from build123d import *

# Parameters (mm, degrees)
PAD_DEPTH       = 20
SKETCH001_R     = 1.5
POCKET_DEPTH    = 50.001
SKETCH002_R     = 2.25
POCKET001_DEPTH = 10.001
SKETCH003_R     = 3.5
POCKET002_DEPTH = 2
PAD001_DEPTH    = 10
SKETCH006_W     = 17
SKETCH006_H     = 7
PAD002_DEPTH    = 36
SKETCH007_W     = 17
SKETCH007_H     = 13
PAD003_DEPTH    = 4
FILLET_R        = 3.5
FILLET001_R     = 3.5
FILLET002_R     = 6
FILLET003_R     = 6
FILLET004_R     = 5
FILLET005_R     = 5
FILLET006_R     = 5
FILLET007_R     = 2
FILLET008_R     = 2
POCKET003_START = -3
SKETCH008_W     = 1.5
SKETCH008_H     = 7
POCKET003_DEPTH = 32


with BuildPart() as part:
    # Sketch → Pad (new body)
    with BuildSketch(Plane.XY):
        Polygon((0, 50), (0, 0), (178, 0), (178, 10), (10, 10), (10, 50), align=None)
    extrude(amount=PAD_DEPTH)

    # Sketch001 (on Face2 of Pad) → Pocket (cut, through all)
    with BuildSketch(Plane.XZ):
        with Locations((117.5, 10)):
            Circle(SKETCH001_R)
        with Locations((167.5, 10)):
            Circle(SKETCH001_R)
    extrude(amount=-POCKET_DEPTH, mode=Mode.SUBTRACT)

    # Sketch002 (on Face6 of Pocket) → Pocket001 (cut, through all)
    with BuildSketch(Plane.YZ.offset(10)):
        with Locations((19.428571, 10)):
            Circle(SKETCH002_R)
        with Locations((36.571429, 10)):
            Circle(SKETCH002_R)
    extrude(amount=-POCKET001_DEPTH, mode=Mode.SUBTRACT)

    # Sketch003 (on Face5 of Pocket001) → Pocket002 (cut)
    with BuildSketch(Plane.XZ):
        with Locations((117.5, 10)):
            Circle(SKETCH003_R)
        with Locations((167.5, 10)):
            Circle(SKETCH003_R)
    extrude(amount=-POCKET002_DEPTH, mode=Mode.SUBTRACT)

    # Sketch004 (on Face10 of Pocket002) → Pad001 (join)
    with BuildSketch(Plane(origin=(0, 10, 0), x_dir=(-1, 0, 0), z_dir=(0, 1, 0))):
        Polygon((-35.5, 20), (-35.5, 51.5), (-52.5, 51.5), (-178, 20), (-149.246042, 20), (-52.5, 44.282871), (-52.5, 20), align=None)
        Polygon((-52.5, 0), (-52.5, -24.282871), (-149.246042, 0), (-178, 0), (-52.5, -31.5), (-35.5, -31.5), (-35.5, 0), align=None)
    extrude(amount=-PAD001_DEPTH)

    # Sketch006 (on Face15 of Pad001) → Pad002 (join)
    with BuildSketch(Plane.XZ):
        with Locations((44, 55)):
            Rectangle(SKETCH006_W, SKETCH006_H)
        with Locations((44, -35)):
            Rectangle(SKETCH006_W, SKETCH006_H)
    extrude(amount=-PAD002_DEPTH)

    # Sketch007 (on Face31 of Pad002) → Pad003 (join)
    with BuildSketch(Plane(origin=(0, 36, 0), x_dir=(-1, 0, 0), z_dir=(0, 1, 0))):
        with Locations((-44, -32)):
            Rectangle(SKETCH007_W, SKETCH007_H)
        with Locations((-44, 52)):
            Rectangle(SKETCH007_W, SKETCH007_H)
    extrude(amount=PAD003_DEPTH)

    # Fillet
    fillet_edges = [part.edges().sort_by_distance(p)[0] for p in [
        (44, 40, 45.5),
    ]]
    fillet(fillet_edges, radius=FILLET_R)

    # Fillet001
    fillet001_edges = [part.edges().sort_by_distance(p)[0] for p in [
        (44, 40, -25.5),
    ]]
    fillet(fillet001_edges, radius=FILLET001_R)

    # Fillet002
    fillet002_edges = [part.edges().sort_by_distance(p)[0] for p in [
        (44, 40, 58.5),
    ]]
    fillet(fillet002_edges, radius=FILLET002_R)

    # Fillet003
    fillet003_edges = [part.edges().sort_by_distance(p)[0] for p in [
        (44, 40, -38.5),
    ]]
    fillet(fillet003_edges, radius=FILLET003_R)

    # Fillet004
    fillet004_edges = [part.edges().sort_by_distance(p)[0] for p in [
        (44, 0, -38.5),
    ]]
    fillet(fillet004_edges, radius=FILLET004_R)

    # Fillet005
    fillet005_edges = [part.edges().sort_by_distance(p)[0] for p in [
        (44, 0, 58.5),
    ]]
    fillet(fillet005_edges, radius=FILLET005_R)

    # Fillet006
    fillet006_edges = [part.edges().sort_by_distance(p)[0] for p in [
        (178, 0, 10),
    ]]
    fillet(fillet006_edges, radius=FILLET006_R)

    # Fillet007
    fillet007_edges = [part.edges().sort_by_distance(p)[0] for p in [
        (0, 0, 10),
    ]]
    fillet(fillet007_edges, radius=FILLET007_R)

    # Fillet008
    fillet008_edges = [part.edges().sort_by_distance(p)[0] for p in [
        (0, 50, 10),
    ]]
    fillet(fillet008_edges, radius=FILLET008_R)

    # Sketch008 (on Face8 of Fillet008) → Pocket003 (cut)
    with BuildSketch(Plane(origin=(35.5, 0, 0), x_dir=(0, -1, 0), z_dir=(-1, 0, 0)).offset(POCKET003_START)):
        with Locations((-9.25, 43.5)):
            Rectangle(SKETCH008_W, SKETCH008_H)
        with Locations((-9.25, -23.5)):
            Rectangle(SKETCH008_W, SKETCH008_H)
    extrude(amount=-POCKET003_DEPTH, mode=Mode.SUBTRACT)


solid = part.part
Build history of the part. All positions in model axes, mm. A direction names the side the tool comes from. Give positions to 0.01 mm unless a question says otherwise; leave off trailing zeros. Order: outer loops, then holes, each group sorted by start corner. A loop starts at its lowest first (then second) coordinate and runs counter-clockwise, first axis right, second up. Notation, with made-up numbers: M -37.5,59 L -1.5,59 A15 ccw -1.5,71 Z; hole C -2.5,-10 d10. An arc over 180 degrees is marked long. Put each result on its own line as item: value.
Item 1: Slice it at A-A, the plane y = 24. Write the cut outline in (x, z), plus the area to 3 significant figures.
From the geometry:
outline: M 0,0 L 10,0 L 10,20 L 0,20 Z; M 35.5,-38.5 L 52.5,-38.5 L 52.5,-31.5 L 35.5,-31.5 Z; M 35.5,51.5 L 52.5,51.5 L 52.5,58.5 L 35.5,58.5 Z
area: 438 mm2
Item 2: Slice it at B-B, the plane z = 36. Write the cut outline in (x, y).
From the geometry:
outline: M 35.5,0 L 52.5,0 L 52.5,10 L 35.5,10 Z; M 85.5,0 L 114.25,0 L 114.25,10 L 85.5,10 Z
Item 3: Slice it at D-D, the plane x = 25. Write the cut outline in (y, z), plus the area to 3 significant figures.
From the geometry:
outline: M 0,0 L 10,0 L 10,20 L 0,20 Z
area: 200 mm2
Item 4: Two-plate mould, pull along X, no slides. Class faces 1 (the flat face through (52.5, 5, -12)), 2 (the cylindrical face through (44.12, 1.43, 57)), 3 (the flat face through (101.55, 5.07, 31.97)), 4 (the flat face through (52.5, 20, -35)): +X half, -X half, draft (parallel to the pull), parting line (faces both ways), or undercut.
From the geometry:
face 1: undercut
face 2: draft
face 3: undercut
face 4: +X half
Item 5: Flat gauge pins, fed straight in: pin 1 Ø4 at (y, z) = (20, 54) entering from +X; pin 2 Ø6 at (x, y) = (61.5, 8) entering from -Z; pin 3 Ø10 at (x, y) = (64, 10.5) entering from -Z; pin 4 Ø10 at (x, y) = (35, 27) entering from -Z. Where does each tip first touch, or does it go through?
From the geometry:
pin 1: stops at x = 52.5
pin 2: stops at z = -29.99
pin 3: stops at z = -29.86
pin 4: stops at z = -38.5
Item 6: 3-axis set-ups, long thin cutter, end or side, ignore diameter. For faces 5 (the flat face through (100, 5, 0)), 6 (the flat face through (44, 36, 49)), 7 (the flat face through (9.6, 19.8, 20)): which of +Z, -Z, +X, -X, +Y, -Y reach the whole face in a straight line?
From the geometry:
face 5: +Y, -Y
face 6: +X, -X
face 7: +Z, -X, +Y, -Y
Item 7: Slice it at C-C, the plane x = 145. Write the cut outline in (y, z).
From the geometry:
outline: M 0,-8.28 L 10,-8.28 L 10,-1.07 L 0,-1.07 Z; M 0,0 L 10,0 L 10,20 L 0,20 Z; M 0,21.07 L 10,21.07 L 10,28.28 L 0,28.28 Z
Item 8: Probe line 1 (Z direction, x = 117.5, y = 0.95); line 2 (Y direction, x = 48.5, z = 28); line 3 (Z direction, x = 74.5, y = 3). List the from-to ranges inside material, lowest first. Write a range as [from, to].
From the geometry:
line 1: z = [-15.19, -7.97], [0, 6.5], [13.5, 20], [27.97, 35.19]
line 2: y = [0, 10]
line 3: z = [-25.98, -18.76], [0, 20], [38.76, 45.98]
